Work out the finished part from the listing and answer in its coordinate system (mm). A direction names the side the tool comes from. Coordinates: 2 decimals unless noted, no trailing zeros. Loops run counter-clockwise (first coordinate to the right, second up) from the corner with the lowest first, then second, coordinate; pieces in that order, holes last.
```python
from build123d import *

# Parameters (mm, degrees)
SZKIC1_R                    = 2
DODANIE_WYCI_GNI_CIE1_DEPTH = 12
SZKIC2_R                    = 3
DODANIE_WYCI_GNI_CIE2_DEPTH = 2
WYTNIJ_WYCI_GNI_CIE1_DEPTH  = 1


with BuildPart() as part:
    # Szkic1 → Dodanie-wyciągnięcie1 (new body)
    with BuildSketch(Plane.XY):
        Circle(SZKIC1_R)
    extrude(amount=DODANIE_WYCI_GNI_CIE1_DEPTH)

    # Szkic2 → Dodanie-wyciągnięcie2 (add)
    with BuildSketch(Plane.XY.offset(12)):
        Circle(SZKIC2_R)
    extrude(amount=DODANIE_WYCI_GNI_CIE2_DEPTH)

    # Szkic3 → Wytnij-wyciągnięcie1 (cut)
    with BuildSketch(Plane.XY.offset(14)):
        Polygon((0.466528249, 0.5), (2, 0.5), (2, -0.5), (0.466528249, -0.5), (0.466528249, -2), (-0.533471751, -2), (-0.533471751, -0.5), (-2, -0.5), (-2, 0.5), (-0.533471751, 0.5), (-0.533471751, 2), (0.466528249, 2), align=None)
    extrude(amount=-WYTNIJ_WYCI_GNI_CIE1_DEPTH, mode=Mode.SUBTRACT)


solid = part.part
```
1. Straight lines are drawn through the part: probe 1 along Z at (x, y) = (0.2, 2.7); probe 2 along Z at (x, y) = (-0.25, -1.7); probe 3 along X at (y, z) = (-1.1, 7). For each, find the intervals that lie inside material, in ascending order.
2. Each of these flat-tipped pins is pushed along its axis until it touches: P1, Ø0.5, axis at y = -1.5, z = 13.5, coming from the -X side; P2, Ø0.8, axis at y = -1.5, z = 13.5, coming from the +X side; P3, Ø0.8, axis at x = -1, z = 13.5, coming from the +Y side. Where does it stop, or does it pass through?
3. A cutting plane is placed at C-C, the plane z = 3.75. Give the vertices of the cut face in (x, y).
4. Determine the mould class of faces 1 (the cylindrical face through (-3, 0, 13)), 2 (the flat face through (0, -2, 13.5)), 3 (the flat face through (1.2, 0.5, 13.5)), 4 (the flat face through (1, -1, 14)) for opening direction Y: released by +Y, released by -Y, zero draft, split by the parting line, or undercut.
5. For faces 5 (the flat face through (-0.533, 1.2, 13.5)), 6 (the cylindrical face through (0, -2, 6)), 7 (the flat face through (0, 0, 0)), determine the directions among +Z, -Z, +X, -X, +Y, -Y from which every point of the face is accessible in a straight line to the end or side of a thin tool.
6. A cutting plane is placed at D-D, the plane y = -2.5. Give the vertices of the cut face in (x, z), then the cut area to 3 significant figures.
7. A cutting plane is placed at A-A, the plane x = 0. Give the vertices of the cut face in (y, z).
Answers below:
1. probe 1: z = 12 to 14
1. probe 2: z = 0 to 13
1. probe 3: x = -1.67 to 1.67
2. P1: stops at x = -2.73
2. P2: stops at x = 2.79
2. P3: stops at y = 2.94
3. outline: circle Ø4 at (0, 0)
4. face 1: split by the parting line
4. face 2: undercut
4. face 3: undercut
4. face 4: zero draft
5. face 5: +Z
5. face 6: -Z
5. face 7: -Z, +X, -X, +Y, -Y
6. outline: (-1.66, 12) - (1.66, 12) - (1.66, 14) - (-1.66, 14) - close
6. area: 6.63 mm2
7. outline: (-3, 12) - (-2, 12) - (-2, 0) - (2, 0) - (2, 12) - (3, 12) - (3, 14) - (2, 14) - (2, 13) - (-2, 13) - (-2, 14) - (-3, 14) - close
